Verification items for the finished model (mm, model axes). Round coordinates to 2 decimals unless told otherwise and drop trailing zeros. Order: outer loops, then holes, each group sorted by start corner. A loop starts at its lowest first (then second) coordinate and runs counter-clockwise, first axis right, second up. Notation, with made-up numbers: (80.5, -7) -> (92.5, -7) arc R36 cw to (92.5, 31) -> close; hole circle Ø3 at (9.5, 89). An arc over 180 degrees is marked (long way). Return JSON: item names as keys, results as strings. Group by question number.
1) Section check A-A on z = 5. Enter the section's corners in (x, y), plus the area to 3 significant figures.
2) Depth check by flat-ended pin: pin 1 (2.5 mm diameter, centred on x = 13, z = 5, fed in from -Y). Enter the tip coordinate at first touch or a pass-through.
3) Scan lines: L1, parallel to X at y = 7.5, z = 5; L2, parallel to Z at x = 13, y = 1.5; L3, parallel to X at y = 8.5, z = 5.5. Record each from-to range of solid material in increasing order.
4) Section check C-C on x = 45. Enter the section's corners in (y, z).
5) Section check B-B on y = 3.5. Enter the section's corners in (x, z), plus the area to 3 significant figures.
6) Draft check along Z on faces 1 (the flat face through (29, -5, 5)), 2 (the flat face through (29, 3, 0)), 3 (the cylindrical face through (11.4, 3.1, 6.2)), 4 (the flat face through (29, 3, 10)). Enter one of: pulls with the +Z half, pulls with the -Z half, needs draft (parallel to the pull), parting line crosses it, or undercut.
Autodesk Inventor part; units mm, degrees
ref_plane "YZ Plane" through (0, 0, 0) normal (1, 0, 0) x (0, 1, 0)
ref_plane "XZ Plane" through (0, 0, 0) normal (0, 1, 0) x (-1, 0, 0)
ref_plane "XY Plane" through (0, 0, 0) normal (0, 0, 1) x (1, 0, 0)
sketch "Sketch1" plane through (0, 0, 0) normal (0, 0, 1) x (1, 0, 0)
  line L0 (50, -5) -> (50, 11)
  line L1 (50, 11) -> (8, 11)
  line L2 (8, -5) -> (8, 11)
  line L3 (8, -5) -> (50, -5)
  dimension "d1" = 16
  dimension "d47" = 42
extrude "Extrusion3" add sketch "Sketch1" along normal blind 10
sketch "Sketch6" plane through (8, 11, 0) normal (0, 1, 0) x (1, 0, 0)
  circle A0 centre (5, -5) radius 2
  circle A1 centre (37, -5) radius 2
  line L0 (42, 0) -> (0, 0)
  line L1 (42, 0) -> (42, -10)
  line L2 (0, 0) -> (0, -10)
  dimension "d48" = 4
  dimension "d49" = 4
  dimension "d50" = 5
  dimension "d51" = 5
  dimension "d52" = 5
  dimension "d53" = 5
extrude "Extrusion7" cut sketch "Sketch6" against normal blind 50
properties part number "Espaciador Sub Inferior" material "Aluminum 6061"
Check result:
{
 "1": {"outline": "(8, -5) -> (11, -5) -> (11, 11) -> (8, 11) -> close; (15, -5) -> (43, -5) -> (43, 11) -> (15, 11) -> close; (47, -5) -> (50, -5) -> (50, 11) -> (47, 11) -> close", "area": "544 mm^2"},
 "2": {"pin 1": "through"},
 "3": {"L1": "8 to 11, 15 to 43, 47 to 50", "L2": "0 to 3, 7 to 10", "L3": "8 to 11.06, 14.94 to 43.06, 46.94 to 50"},
 "4": {"outline": "(-5, 0) -> (11, 0) -> (11, 3) -> (-5, 3) -> close; (-5, 7) -> (11, 7) -> (11, 10) -> (-5, 10) -> close"},
 "5": {"outline": "(8, 0) -> (50, 0) -> (50, 10) -> (8, 10) -> close; hole circle Ø4 at (13, 5); hole circle Ø4 at (45, 5)", "area": "395 mm^2"},
 "6": {"face 1": "needs draft", "face 2": "pulls with the -Z half", "face 3": "undercut", "face 4": "pulls with the +Z half"}
}
